Geometry check sheet. Reference: the model listing, model coordinates, mm. Face numbers are marked on the shaded views. Give positions to 0.01 mm unless a question says otherwise; leave off trailing zeros. Order: outer loops, then holes, each group sorted by start corner. A loop starts at its lowest first (then second) coordinate and runs counter-clockwise, first axis right, second up.
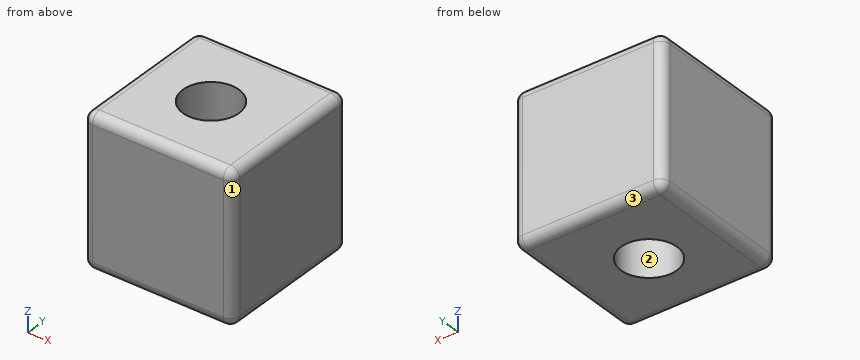
from build123d import *

# Parameters (mm, degrees)
F0_W     = 80
F0_H     = 80
F1_DEPTH = 80
F2_R     = 15
F3_DEPTH = 80.001
F4_R     = 5


with BuildPart() as f1:
    # F0 (on Top) → F1 (new body)
    with BuildSketch(Plane.XY):
        with Locations((1.3716, 17.491502)):
            Rectangle(F0_W, F0_H)
    extrude(amount=F1_DEPTH)

    # F2 (on face) → F3 (cut, through all)
    with BuildSketch(Plane.XY.offset(80)):
        with Locations((0, 16.490143)):
            Circle(F2_R)
    extrude(amount=-F3_DEPTH, mode=Mode.SUBTRACT)

    # F4
    f4_edges = [f1.edges().sort_by_distance(p)[0] for p in [
        (1.3716, 57.491502, 80),
        (1.3716, -22.508498, 80),
        (-38.6284, 17.491502, 80),
        (41.3716, 17.491502, 80),
        (41.3716, 57.491502, 40),
        (41.3716, -22.508498, 40),
        (41.3716, 17.491502, 0),
        (-38.6284, 57.491502, 40),
        (-38.6284, 17.491502, 0),
        (-38.6284, -22.508498, 40),
        (1.3716, 57.491502, 0),
        (1.3716, -22.508498, 0),
    ]]
    fillet(f4_edges, radius=F4_R)


solid = f1.part
Item 1: Draft check along Y on the marked faces 1, 2 and 3. Enter one of: released by +Y, released by -Y, zero draft, split by the parting line, or undercut.
Reported:
face 1: released by -Y
face 2: undercut
face 3: released by +Y
Item 2: Scan lines: L1, parallel to Y at x = 0, z = 25; L2, parallel to X at y = 17, z = 56; L3, parallel to X at y = 13.5, z = 37.5. Record each from-to range of solid material in increasing order.
Reported:
L1: y = -22.51 to 1.49, 31.49 to 57.49
L2: x = -38.63 to -14.99, 14.99 to 41.37
L3: x = -38.63 to -14.7, 14.7 to 41.37
Item 3: Sectioned sample at B-B (z = 56). Enter the section's corners in (x, y), and give its area (3 significant figures).
Reported:
outline: (-38.63, -17.51) arc R5 ccw to (-33.63, -22.51) - (36.37, -22.51) arc R5 ccw to (41.37, -17.51) - (41.37, 52.49) arc R5 ccw to (36.37, 57.49) - (-33.63, 57.49) arc R5 ccw to (-38.63, 52.49) - close; hole circle Ø30 at (0, 16.49)
area: 5,670 mm2
Item 4: Sectioned sample at A-A (x = 0). Enter the section's corners in (y, z).
Reported:
outline: (-22.51, 5) arc R5 ccw to (-17.51, 0) - (1.49, 0) - (1.49, 80) - (-17.51, 80) arc R5 ccw to (-22.51, 75) - close; (31.49, 0) - (52.49, 0) arc R5 ccw to (57.49, 5) - (57.49, 75) arc R5 ccw to (52.49, 80) - (31.49, 80) - close
Item 5: Sectioned sample at C-C (y = 27.5). Enter the section's corners in (x, z), and give its area (3 significant figures).
Reported:
outline: (-38.63, 5) arc R5 ccw to (-33.63, 0) - (-10.19, 0) - (-10.19, 80) - (-33.63, 80) arc R5 ccw to (-38.63, 75) - close; (10.19, 0) - (36.37, 0) arc R5 ccw to (41.37, 5) - (41.37, 75) arc R5 ccw to (36.37, 80) - (10.19, 80) - close
area: 4,750 mm2
